Can you work these out from the model? Positions are in its coordinate system, mm. Face numbers are marked on the shaded views. Coordinates: 2 decimals unless noted, no trailing zeros. Order: outer loops, then holes, each group sorted by start corner. A loop starts at its lowest first (then second) coordinate and runs counter-clockwise, first axis right, second up. Notation, with made-up numbers: (-10.5, -26.75) -> (21.5, -26.75) arc R19 ccw to (21.5, -10.75) -> close; hole circle Ø1 at (13, 33.25). An arc over 180 degrees is marked (long way). Use a Markdown table: item, result. Add a question column.
1. For pin 1 Ø8 at (x, y) = (-23.55, -23.55) entering from +Z, with a flat end and sliding along its axis, tell me the tip position at first contact or that it passes through.
2. Suppose I cut it at C-C, the plane y = -39. State how many separate pieces and enclosed holes the cut face has, then the cut area to 3 significant figures.
3. We'd pull the mould along X, two halves only. Please class the marked faces 1 and 2: pulls with the +X half, pulls with the -X half, needs draft (parallel to the pull), parting line crosses it, or undercut.
4. Suppose I cut it at D-D, the plane x = -37.5. List the corners of the cut face in (y, z) for me.
5. Suppose I cut it at B-B, the plane z = 93.5. List the corners of the cut face in (x, y) for me.
6. Suppose I cut it at A-A, the plane y = 23.55. List the corners of the cut face in (x, z) for me.
7. If I drill on line 1 along Y through (x, z) = (23.55, 3.8); line 2 along Y through (x, z) = (-33, 159); line 3 along Z through (x, y) = (32, 39), over which ranges is the centre line in solid material (lowest first)? Write a range as from..to.
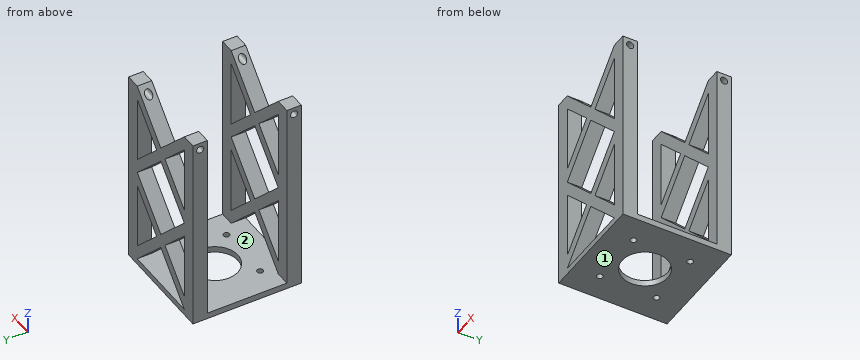
```python
from build123d import *

# Parameters (mm, degrees)
F0_W      = 90
F0_H      = 90
F0_R      = 2.5
F0_R_2    = 19
F1_DEPTH  = 5
F3_W      = 12
F3_H      = 12
F4_DEPTH  = 160
F7_DEPTH  = 12
F10_DEPTH = 12
F12_R     = 3
F13_DEPTH = 90.001


with BuildPart() as f1:
    # F0 (on Top) → F1 (new body)
    with BuildSketch(Plane.XY):
        Rectangle(F0_W, F0_H)
        with Locations((-23.55, -23.55)):
            Circle(F0_R, mode=Mode.SUBTRACT)
        with Locations((23.55, -23.55)):
            Circle(F0_R, mode=Mode.SUBTRACT)
        with Locations((-23.55, 23.55)):
            Circle(F0_R, mode=Mode.SUBTRACT)
        Circle(F0_R_2, mode=Mode.SUBTRACT)
        with Locations((23.55, 23.55)):
            Circle(F0_R, mode=Mode.SUBTRACT)
    extrude(amount=F1_DEPTH)

    # F3 (on offset) → F4 (join)
    with BuildSketch(Plane.XY.offset(5)):
        with Locations((-39, -39)):
            Rectangle(F3_W, F3_H)
        with Locations((39, -39)):
            Rectangle(F3_W, F3_H)
        with Locations((39, 39)):
            Rectangle(F3_W, F3_H)
        with Locations((-39, 39)):
            Rectangle(F3_W, F3_H)
    extrude(amount=F4_DEPTH)

    # F6 (on offset) → F7 (join)
    with BuildSketch(Plane.XZ.offset(45)):
        Polygon((0, 51), (5.8235294118, 45), (33, 73), (33, 85), align=None)
        Polygon((0, 119), (33, 85), (33, 97), (5.8235294118, 125), align=None)
        Polygon((0, 131), (5.8235294118, 125), (33, 153), (33, 165), align=None)
        Polygon((-33, 153), (-5.8235294118, 125), (0, 131), (-33, 165), align=None)
        Polygon((-33, 97), (-33, 85), (0, 119), (-5.8235294118, 125), align=None)
        Polygon((-5.8235294118, 125), (0, 119), (5.8235294118, 125), (0, 131), align=None)
        Polygon((-5.8235294118, 45), (0, 39), (5.8235294118, 45), (0, 51), align=None)
        Polygon((-33, 73), (-5.8235294118, 45), (0, 51), (-33, 85), align=None)
        Polygon((-33, 17), (-33, 5), (0, 39), (-5.8235294118, 45), align=None)
        Polygon((5.8235294118, 45), (0, 39), (33, 5), (33, 17), align=None)
    extrude(amount=-F7_DEPTH)

    # F9 (on offset) → F10 (join)
    with BuildSketch(Plane(origin=(0, 45, 0), x_dir=(-1, 0, 0), z_dir=(0, 1, 0))):
        Polygon((-33, 153), (-5.8235294118, 125), (0, 131), (-33, 165), align=None)
        Polygon((-5.8235294118, 125), (0, 119), (5.8235294118, 125), (0, 131), align=None)
        Polygon((0, 131), (5.8235294118, 125), (33, 153), (33, 165), align=None)
        Polygon((0, 119), (33, 85), (33, 97), (5.8235294118, 125), align=None)
        Polygon((-33, 85), (0, 119), (-5.8235294118, 125), (-33, 97), align=None)
        Polygon((-5.8235294118, 45), (0, 51), (-33, 85), (-33, 73), align=None)
        Polygon((0, 39), (-5.8235294118, 45), (-33, 17), (-33, 5), align=None)
        Polygon((33, 73), (33, 85), (0, 51), (5.8235294118, 45), align=None)
        Polygon((33, 17), (5.8235294118, 45), (0, 39), (33, 5), align=None)
        Polygon((5.8235294118, 45), (0, 51), (-5.8235294118, 45), (0, 39), align=None)
    extrude(amount=-F10_DEPTH)

    # F12 (on offset) → F13 (cut, through all)
    with BuildSketch(Plane.YZ.offset(45)):
        with Locations((-39, 159)):
            Circle(F12_R)
        with Locations((39, 159)):
            Circle(F12_R)
    extrude(amount=-F13_DEPTH, mode=Mode.SUBTRACT)


solid = f1.part
```
Worked out:
| question | item | result |
|---|---|---|
| 1 | pin 1 | stops at z = 5 |
| 2 | separate pieces | 3 |
| 2 | enclosed holes | 6 |
| 2 | area | 7,100 mm² |
| 3 | face 1 | needs draft |
| 3 | face 2 | undercut |
| 4 | outline | (-45, 0) -> (45, 0) -> (45, 165) -> (33, 165) -> (33, 5) -> (-33, 5) -> (-33, 165) -> (-45, 165) -> close; hole circle Ø6 at (-39, 159); hole circle Ø6 at (39, 159) |
| 5 | outline | (-45, -45) -> (-24.75, -45) -> (-24.75, -33) -> (-45, -33) -> close; (-45, 33) -> (-24.75, 33) -> (-24.75, 45) -> (-45, 45) -> close; (24.75, -45) -> (45, -45) -> (45, -33) -> (24.75, -33) -> close; (24.75, 33) -> (45, 33) -> (45, 45) -> (24.75, 45) -> close |
| 6 | outline | (-45, 0) -> (-26.05, 0) -> (-26.05, 5) -> (-45, 5) -> close; (-21.05, 0) -> (21.05, 0) -> (21.05, 5) -> (-21.05, 5) -> close; (26.05, 0) -> (45, 0) -> (45, 5) -> (26.05, 5) -> close |
| 7 | line 1 | y = -45..-26.05, -21.05..21.05, 26.05..45 |
| 7 | line 2 | y = -45..-42, -36..-33, 33..36, 42..45 |
| 7 | line 3 | z = 0..5, 6.03..18.03, 71.97..83.97, 86.03..98.03, 151.97..156, 162..163.97 |
